The listing builds one solid part. Answer for the finished solid, in the listing's coordinates (mm). Face numbers are marked on the shaded views. A direction names the side the tool comes from. Give positions to 0.01 mm unless a question says otherwise; leave off trailing zeros. Write each question's results on one line, items separated by ' | '. Start each with the question number.
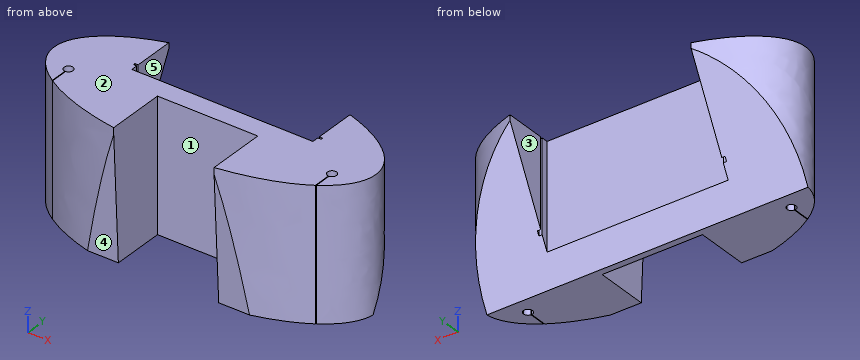
from build123d import *

# Parameters (mm, degrees)
SKETCH1_RX               = 244
SKETCH1_RY               = 110
BOSS_EXTRUDE1_DEPTH      = 200
SKETCH12_R               = 6.83635542
CUT_EXTRUDE8_DEPTH       = 201
CUT_EXTRUDE10_DEPTH      = 245
CUT_EXTRUDE10_DEPTH_BACK = 245
CUT_EXTRUDE11_DEPTH      = 1.0000001
CUT_EXTRUDE11_DEPTH_BACK = 201.0000001
SKETCH17_W               = 152.4
SKETCH17_H               = 90
CUT_EXTRUDE12_DEPTH      = 1.0000001
CUT_EXTRUDE12_DEPTH_BACK = 201.0000001
SKETCH18_W               = 1
SKETCH18_H               = 33.332943991
CUT_EXTRUDE13_DEPTH      = 1.0000001
CUT_EXTRUDE13_DEPTH_BACK = 201.0000001


with BuildPart() as part:
    # Sketch1 → Boss-Extrude1 (new body)
    with BuildSketch(Plane.XY):
        with Locations((0, 0)):
            Ellipse(SKETCH1_RX, SKETCH1_RY)
    extrude(amount=-BOSS_EXTRUDE1_DEPTH)

    # Sketch12 → Cut-Extrude8 (cut, through all)
    with BuildSketch(Plane.XY):
        with Locations((200, -30)):
            Circle(SKETCH12_R)
        with Locations((-200, -30)):
            Circle(SKETCH12_R)
    extrude(amount=-CUT_EXTRUDE8_DEPTH, mode=Mode.SUBTRACT)

    # Sketch15 → Cut-Extrude10 (cut, two sides)
    with BuildSketch(Plane(origin=(0, 0, 0), x_dir=(0, 0, -1), z_dir=(1, 0, 0))) as cut_extrude10_sk:
        Polygon((0, 110), (0, 95), (200, -5), (200, 110), align=None)
        Polygon((0, -110), (200, -110), (200, -95), (0, -105), align=None)
    extrude(amount=CUT_EXTRUDE10_DEPTH, mode=Mode.SUBTRACT)
    extrude(cut_extrude10_sk.sketch, amount=-CUT_EXTRUDE10_DEPTH_BACK, mode=Mode.SUBTRACT)

    # Sketch16 → Cut-Extrude11 (cut, two sides)
    with BuildSketch(Plane.XY) as cut_extrude11_sk:
        Polygon((-137.5, 95), (137.5, 95), (137.5, 28.1), (142.5, 28.1), (142.5, 25.1), (137.5, 25.1), (137.5, 15.1), (-137.5, 15.1), (-137.5, 25.1), (-142.5, 25.1), (-142.5, 28.1), (-137.5, 28.1), align=None)
    extrude(amount=CUT_EXTRUDE11_DEPTH, mode=Mode.SUBTRACT)
    extrude(cut_extrude11_sk.sketch, amount=-CUT_EXTRUDE11_DEPTH_BACK, mode=Mode.SUBTRACT)

    # Sketch17 → Cut-Extrude12 (cut, two sides)
    with BuildSketch(Plane.XY) as cut_extrude12_sk:
        with Locations((0, -60)):
            Rectangle(SKETCH17_W, SKETCH17_H)
    extrude(amount=CUT_EXTRUDE12_DEPTH, mode=Mode.SUBTRACT)
    extrude(cut_extrude12_sk.sketch, amount=-CUT_EXTRUDE12_DEPTH_BACK, mode=Mode.SUBTRACT)

    # Sketch18 → Cut-Extrude13 (cut, two sides)
    with BuildSketch(Plane.XY) as cut_extrude13_sk:
        with Locations((200, -46.666471996)):
            Rectangle(SKETCH18_W, SKETCH18_H)
        with Locations((-200, -46.666471996)):
            Rectangle(SKETCH18_W, SKETCH18_H)
    extrude(amount=CUT_EXTRUDE13_DEPTH, mode=Mode.SUBTRACT)
    extrude(cut_extrude13_sk.sketch, amount=-CUT_EXTRUDE13_DEPTH_BACK, mode=Mode.SUBTRACT)


solid = part.part
1. Consider probe 1 along X at (y, z) = (-30, -71); probe 2 along X at (y, z) = (-25, -40); probe 3 along Y at (x, z) = (35, -144.5). Determine where each line is inside the solid, lowest interval first. Write a range as [from, to].
2. Each of these flat-tipped pins is pushed along its axis until it touches: pin 1 Ø1.5 at (x, z) = (140.5, -47) entering from +Y (3 decimals); pin 2 Ø3 at (x, z) = (67.5, -102) entering from +Y; pin 3 Ø20.5 at (y, z) = (-49, -140.5) entering from +X. Where does it stop, or does it pass through?
3. A tool of negligible diameter and unlimited length cuts with its end or side. For the marked faces 1, 2 and 3, from which of +Z, -Z, +X, -X, +Y, -Y can it reach the whole face along a straight path? Write none if from no direction.
4. The mould has two halves that part along X. Classify the marked faces 4 and 5: pulls with the +X half, pulls with the -X half, needs draft (parallel to the pull), parting line crosses it, or undercut.
Results:
1) probe 1: x = [-234.75, -206.84], [-193.16, -76.2], [76.2, 193.16], [206.84, 234.75] | probe 2: x = [-237.61, -204.66], [-195.34, -76.2], [76.2, 195.34], [204.66, 237.61] | probe 3: y = [-15, 15.1]
2) pin 1: stops at y = 71.875 | pin 2: stops at y = 15.1 | pin 3: stops at x = 228.36
3) face 1: +Z, -Z, -Y | face 2: +Z, +X, -X, +Y, -Y | face 3: +Z, -Z, +Y
4) face 4: needs draft | face 5: undercut
